from build123d import *

# Parameters (mm, degrees)
SKETCH1_R           = 1.4986
SKETCH1_R_2         = 3.556
BOSS_EXTRUDE2_DEPTH = 3.175


with BuildPart() as part:
    # Sketch1 → Boss-Extrude2 (new body)
    with BuildSketch(Plane(origin=(0, 0, 0), x_dir=(1, 0, 0), z_dir=(0, 1, 0))):
        with BuildLine():
            Line((-3.88054086, 24.446655173), (-3.88054086, -2.874238183))
            add(Edge.make_bspline(
                [(-5.126415425, -7.816187942), (-4.308579975, -6.333908563), (-3.879875529, -4.567729194), (-3.88054086, -2.874238183)],
                knots=[2, 2, 2, 2, 3, 3, 3, 3], degree=3))
            add(Edge.make_bspline(
                [(-5.016324889, -13.818322138), (-6.095643591, -12.023073271), (-6.186493664, -9.73551085), (-5.126415425, -7.816187942)],
                knots=[1.005658807, 1.005658807, 1.005658807, 1.005658807, 2, 2, 2, 2], degree=3))
            add(Edge.make_bspline(
                [(-3.88054086, -18.316067774), (-3.88054086, -16.774680236), (-4.271386719, -15.167168465), (-5.016324889, -13.818322138)],
                knots=[17, 17, 17, 17, 18, 18, 18, 18], degree=3))
            Line((-3.88054086, -18.316067774), (-3.991875118, -23.843497505))
            ThreePointArc((-3.991875118, -23.843497505), (0.001069913, -27.836442536), (3.994014944, -23.843497505))
            Line((3.994014944, -23.843497505), (3.994014944, -18.759718562))
            add(Edge.make_bspline(
                [(5.241762742, -13.818322138), (4.423413244, -15.300216615), (3.994014944, -17.066290901), (3.994014944, -18.759718562)],
                knots=[11, 11, 11, 11, 12, 12, 12, 12], degree=3))
            add(Edge.make_bspline(
                [(5.522924723, -7.816187942), (6.529884526, -9.766435102), (6.373924923, -12.053304327), (5.241762742, -13.818322138)],
                knots=[9, 9, 9, 9, 10, 10, 10, 10], degree=3))
            add(Edge.make_bspline(
                [(4.275176926, -2.874728037), (4.275176926, -4.568219179), (4.704575226, -6.334229984), (5.522924723, -7.816187942)],
                knots=[8, 8, 8, 8, 9, 9, 9, 9], degree=3))
            Line((4.275176926, -2.874728037), (4.275176926, 24.479419578))
            ThreePointArc((4.275176926, 24.479419578), (0.180935831, 28.540896268), (-3.88054086, 24.446655173))
        make_face()
        with Locations(Location((0.197318033, 24.463037376, 0), (0, 0, 270))):
            Circle(SKETCH1_R, mode=Mode.SUBTRACT)
        with Locations(Location((0.001040667, -10.913296245, 0), (0, 0, 270))):
            Circle(SKETCH1_R_2, mode=Mode.SUBTRACT)
        with BuildLine():
            Line((0.999301297, -0.813017652), (0.999301297, 4.187201199))
            ThreePointArc((0.999301297, 4.187201199), (0.001069914, 5.185432583), (-0.99716147, 4.187201199))
            Line((-0.99716147, 4.187201199), (-0.99716147, -0.813017652))
            ThreePointArc((-0.99716147, -0.813017652), (0.001069914, -1.811249036), (0.999301297, -0.813017652))
        make_face(mode=Mode.SUBTRACT)
        with BuildLine():
            Line((0.999301296, -24.713674478), (0.999301296, -21.01357972))
            ThreePointArc((0.999301296, -21.01357972), (0.001069913, -20.015348337), (-0.997161471, -21.01357972))
            Line((-0.997161471, -21.01357972), (-0.997161471, -24.713674478))
            ThreePointArc((-0.997161471, -24.713674478), (0.001069913, -25.711905862), (0.999301296, -24.713674478))
        make_face(mode=Mode.SUBTRACT)
    extrude(amount=BOSS_EXTRUDE2_DEPTH)


solid = part.part
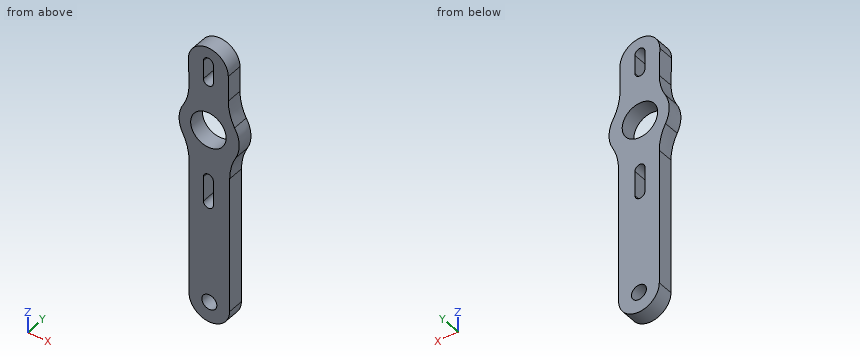
Read the model definition and answer for the solid it produces. Units are mm, in the model's axes. Give positions to 0.01 mm unless a question says otherwise; leave off trailing zeros. Write each loop counter-clockwise with the first axis right and the second up, starting at its lowest first coordinate (ties: lowest second). Pieces come first, ordered by that corner, then holes. Notation, with made-up numbers: (66.5, 15.25) - (122.5, 15.25) arc R33 ccw to (122.5, 52.25) - close; hole circle Ø10 at (28, 66). An arc over 180 degrees is marked (long way). Use CSV: the item, a comma, the result in double quotes. Start each with the question number.
Item 1: The part is cut by section B-B, the plane z = -10. Give the vertices of the cut face in (x, y) (3 decimals).
Item 2: Consider line 1 (Z direction, x = -0.5, y = 0.35); line 2 (Z direction, x = -0.75, y = 3); line 3 (X direction, y = 2.95, z = 23). Determine where each line is inside the solid, lowest interval first.
Item 3: Flat-ended cylindrical pins translate along their axes: P1, Ø1, axis at y = 2, z = 22, coming from the +X side; P2, Ø1.5, axis at y = 2.5, z = 14.5, coming from the -X side; P3, Ø1, axis at y = 2, z = 23, coming from the -X side. Find the tip coordinate at first contact, or state that the pin passes through.
Item 4: The part is cut by section A-A, the plane x = 3. Give the vertices of the cut face in (y, z) (3 decimals).
Item 5: The part is cut by section C-C, the plane y = 0.7. Count the separate pieces of the cut face and the enclosed holes in it, and give its area (3 significant figures).
Taken from the geometry:
1,outline,"(-3.881, 0) - (4.275, 0) - (4.275, 3.175) - (-3.881, 3.175) - close"
2,line 1,"-28.48 to -25.79, -23.14 to -5.05, 1.68 to 7.39, 14.43 to 20.15, 25.58 to 27.8"
2,line 2,"-28.43 to -25.62, -23.3 to -4.84, 1.47 to 7.44, 14.39 to 20.36, 25.37 to 27.77"
2,line 3,"-3.97 to -1, 1 to 3.99"
3,P1,"x = 3.99"
3,P2,"x = -5.06"
3,P3,"x = -3.98"
4,outline,"(0, -27.425) - (3.175, -27.425) - (3.175, 9.002) - (0, 9.002) - close; (0, 12.824) - (3.175, 12.824) - (3.175, 26.48) - (0, 26.48) - close"
5,separate pieces,"1"
5,enclosed holes,"4"
5,area,"400 mm2"
